from build123d import *

# Parameters (mm, degrees)
SKETCH1_R           = 2.4765
BOSS_EXTRUDE1_DEPTH = 9.525
SKETCH2_R           = 3.9624
BOSS_EXTRUDE2_DEPTH = 4.826
CUT_EXTRUDE1_DEPTH  = 2.286
CHAMFER1_SIZE       = 0.508


with BuildPart() as part:
    # Sketch1 → Boss-Extrude1 (new body)
    with BuildSketch(Plane(origin=(0, 0, 0), x_dir=(1, 0, 0), z_dir=(0, 1, 0))):
        with Locations(Location((0, 0, 0), (0, 0, 90))):
            Circle(SKETCH1_R)
    extrude(amount=BOSS_EXTRUDE1_DEPTH)

    # Sketch2 → Boss-Extrude2 (add)
    with BuildSketch(Plane.XZ):
        with Locations(Location((0, 0, 0), (0, 0, 270))):
            Circle(SKETCH2_R)
    extrude(amount=BOSS_EXTRUDE2_DEPTH)

    # Sketch3 → Cut-Extrude1 (cut)
    with BuildSketch(Plane.XZ.offset(4.826)):
        Polygon((2.291358881, 0), (1.14567944, 1.984375), (-1.14567944, 1.984375), (-2.291358881, 0), (-1.14567944, -1.984375), (1.14567944, -1.984375), align=None)
    extrude(amount=-CUT_EXTRUDE1_DEPTH, mode=Mode.SUBTRACT)

    # Chamfer1
    chamfer1_edges = [part.edges().sort_by_distance(p)[0] for p in [
        (0, 0, 3.9624),
        (0, -4.826, 3.9624),
    ]]
    chamfer(chamfer1_edges, length=CHAMFER1_SIZE)


solid = part.part
Source: CAD feature listing. Evaluate the final solid. Frame: model axes, mm. A direction names the side the tool comes from. Round coordinates to 2 decimals unless told otherwise and drop trailing zeros. Loops run counter-clockwise (first coordinate to the right, second up) from the corner with the lowest first, then second, coordinate; pieces in that order, holes last. Notation, with made-up numbers: (31.25, 24) -> (64.25, 24) arc R27 cw to (64.25, 53) -> close; hole circle Ø2 at (60, -20). An arc over 180 degrees is marked (long way). Answer as a JSON object with one key per item and string values. Group by question number.
Q1. Section query B-B (y = 5.5). Output: boundary loops of the cut face in (x, z), plus the area to 3 significant figures.
Q2. Section query A-A (x = 0). Output: boundary loops of the cut face in (y, z) (1 decimal).
Q3. Contact query for flat-ended pins moving along their axis: P1, Ø1, axis at y = 4, z = -2.5, coming from the -X side; P2, Ø1, axis at y = 7.5, z = 2.5, coming from the +X side; P3, Ø2, axis at x = 2, y = 8, coming from the -Z side. Output: stop coordinate, or through.
Q4. Ray query, line 1 (X direction, y = -4, z = 1.25); line 2 (Y direction, x = -2, z = -2); line 3 (Z direction, x = 1.5, y = -4). Return the intervals inside material, ascending. Write a range as from..to.
Q5. Access query for faces 1 (the flat face through (0, -4, 1.984)), 2 (the flat face through (-1.5, 0, -2.3)), 3 (the flat face through (0, 9.525, 0)). Directions: +Z, -Z, +X, -X, +Y, -Y. A direction counts if a zero-diameter tool reaches every point of the face in a straight line with its end or side. Return the directions, or none.
Q6. Mould query, pull axis Z, two halves, no side actions, for faces 4 (the flat face through (2, -4.826, -1)), 5 (the flat face through (0, -2.54, 0)), 6 (the cylindrical face through (-0.744, 4.696, -2.362)), 7 (the flat face through (-1.727, -3.699, -0.978)). Classes: pulls with the +Z half, pulls with the -Z half, needs draft (parallel to the pull), parting line crosses it, or undercut.
Completed:
{
 "1": {"outline": "circle Ø4.95 at (0, 0)", "area": "19.3 mm²"},
 "2": {"outline": "(-4.8, -3.5) -> (-4.3, -4) -> (-0.5, -4) -> (0, -3.5) -> (0, -2.5) -> (9.5, -2.5) -> (9.5, 2.5) -> (0, 2.5) -> (0, 3.5) -> (-0.5, 4) -> (-4.3, 4) -> (-4.8, 3.5) -> (-4.8, 2) -> (-2.5, 2) -> (-2.5, -2) -> (-4.8, -2) -> close"},
 "3": {"P1": "x = -1.46", "P2": "x = 1.46", "P3": "z = -2.27"},
 "4": {"line 1": "-3.76..-1.57, 1.57..3.76", "line 2": "-4.83..0", "line 3": "-3.67..-1.37, 1.37..3.67"},
 "5": {"face 1": "-Y", "face 2": "+Y", "face 3": "+Z, -Z, +X, -X, +Y"},
 "6": {"face 4": "needs draft", "face 5": "undercut", "face 6": "parting line crosses it", "face 7": "undercut"}
}
